The model under review builds one solid part; all positions refer to its coordinate system, in mm. Face numbers are marked on the shaded views. A direction names the side the tool comes from. Round coordinates to 2 decimals unless told otherwise and drop trailing zeros. Order: outer loops, then holes, each group sorted by start corner. A loop starts at its lowest first (then second) coordinate and runs counter-clockwise, first axis right, second up.
```python
from build123d import *

# Parameters (mm, degrees)
SKETCH1_W           = 40.25
SKETCH1_H           = 40
BOSS_EXTRUDE1_DEPTH = 20.25
SKETCH2_R           = 6.5
BOSS_EXTRUDE2_DEPTH = 1.35
SKETCH3_R           = 3
BOSS_EXTRUDE3_DEPTH = 4.25
BOSS_EXTRUDE4_DEPTH = 5.1


with BuildPart() as part:
    # Sketch1 → Boss-Extrude1 (new body)
    with BuildSketch(Plane(origin=(0, 0, 0), x_dir=(1, 0, 0), z_dir=(0, 1, 0))):
        with Locations((20.125, 20)):
            Rectangle(SKETCH1_W, SKETCH1_H)
    extrude(amount=BOSS_EXTRUDE1_DEPTH)

    # Sketch2 → Boss-Extrude2 (add)
    with BuildSketch(Plane.ZY):
        with Locations(Location((-29.5, 10.125, 0), (0, 0, 180))):
            Circle(SKETCH2_R)
    extrude(amount=BOSS_EXTRUDE2_DEPTH)

    # Sketch3 → Boss-Extrude3 (add)
    with BuildSketch(Plane.ZY.offset(1.35)):
        with Locations((-29.5, 10.125)):
            Circle(SKETCH3_R)
    extrude(amount=BOSS_EXTRUDE3_DEPTH)

    # Sketch4 → Boss-Extrude4 (add)
    with BuildSketch(Plane(origin=(12.65, 0, 0), x_dir=(0, 0, -1), z_dir=(1, 0, 0))):
        with BuildLine():
            Line((40, 19.25), (46, 19.25))
            ThreePointArc((46, 19.25), (46.707106781, 18.957106781), (47, 18.25))
            Line((47, 18.25), (47, 15.655745837))
            ThreePointArc((47, 15.655745837), (43.25, 14.6875), (47, 13.719254163))
            Line((47, 13.719254163), (47, 6.530745837))
            ThreePointArc((47, 6.530745837), (43.25, 5.5625), (47, 4.594254163))
            Line((47, 4.594254163), (47, 2))
            ThreePointArc((47, 2), (46.707106781, 1.292893219), (46, 1))
            Line((46, 1), (40, 1))
            Line((40, 1), (40, 19.25))
        make_face()
        with BuildLine():
            Line((0, 19.25), (-6, 19.25))
            ThreePointArc((-6, 19.25), (-6.707106781, 18.957106781), (-7, 18.25))
            Line((-7, 18.25), (-7, 15.655745837))
            ThreePointArc((-7, 15.655745837), (-3.25, 14.6875), (-7, 13.719254163))
            Line((-7, 13.719254163), (-7, 6.530745837))
            ThreePointArc((-7, 6.530745837), (-3.25, 5.5625), (-7, 4.594254163))
            Line((-7, 4.594254163), (-7, 2))
            ThreePointArc((-7, 2), (-6.707106781, 1.292893219), (-6, 1))
            Line((-6, 1), (0, 1))
            Line((0, 1), (0, 19.25))
        make_face()
    extrude(amount=-BOSS_EXTRUDE4_DEPTH)


solid = part.part
```
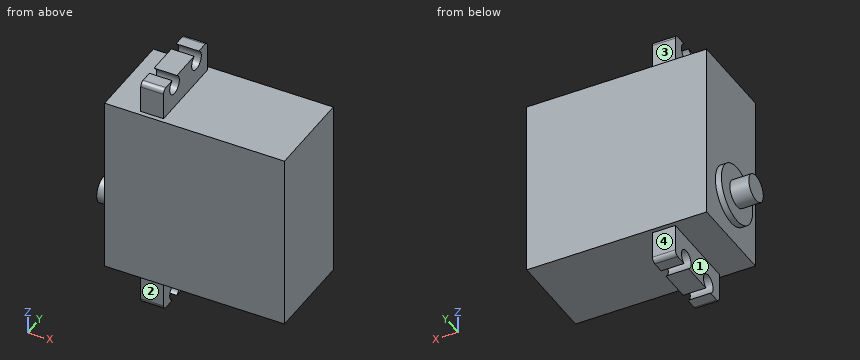
(1) Consider section D-D (x = 35). Write out the cut boundary in (y, z).
Data:
outline: (0, -40) - (20.25, -40) - (20.25, 0) - (0, 0) - close
(2) Insertion check: pin 1 (2.5 mm diameter, centred on x = 10, z = 2.5, fed in from -Y); pin 2 (6 mm diameter, centred on y = 10.5, z = -11, fed in from -X); pin 3 (10 mm diameter, centred on x = -1, y = 6.5, fed in from +Z). Each pin has a flat end and moves straight along its axis. Give the tip position at first contact, or say it passes through.
Data:
pin 1: stops at y = 1
pin 2: stops at x = 0
pin 3: stops at z = 0
(3) Consider section A-A (z = 5.25). Write out the cut boundary in (x, y).
Data:
outline: (7.55, 1) - (12.65, 1) - (12.65, 3.56) - (7.55, 3.56) - close; (7.55, 7.56) - (12.65, 7.56) - (12.65, 12.69) - (7.55, 12.69) - close; (7.55, 16.69) - (12.65, 16.69) - (12.65, 19.25) - (7.55, 19.25) - close
(4) Consider section C-C (y = 9.25). Write out the cut boundary in (x, z), and give its area (3 significant figures).
Data:
outline: (-5.6, -32.37) - (-1.35, -32.37) - (-1.35, -35.94) - (0, -35.94) - (0, -40) - (7.55, -40) - (7.55, -47) - (12.65, -47) - (12.65, -40) - (40.25, -40) - (40.25, 0) - (12.65, 0) - (12.65, 7) - (7.55, 7) - (7.55, 0) - (0, 0) - (0, -23.06) - (-1.35, -23.06) - (-1.35, -26.63) - (-5.6, -26.63) - close
area: 1,720 mm2
(5) For the marked faces 1, 2, 3 and 4, list the 3-axis set-ups (+Z, -Z, +X, -X, +Y, -Y) from which the entire face can be reached by the end or side of a thin tool; tool diameter is ignored.
Data:
face 1: -Z, -X, +Y, -Y
face 2: -Z, +X, -X, -Y
face 3: +Z, +X, -X, +Y
face 4: -Z, +X, -X, +Y
(6) Consider section B-B (z = -29.5). Write out the cut boundary in (x, y) (3 decimals).
Data:
outline: (-5.6, 7.125) - (-1.35, 7.125) - (-1.35, 3.625) - (0, 3.625) - (0, 0) - (40.25, 0) - (40.25, 20.25) - (0, 20.25) - (0, 16.625) - (-1.35, 16.625) - (-1.35, 13.125) - (-5.6, 13.125) - close
(7) To check wall thickness, follow probe 1 along Y at (x, z) = (11.65, -45.25); probe 2 along Y at (x, z) = (10, 5); probe 3 along Z at (x, y) = (36.5, 6). State the ranges of each line that lie inside material, in increasing order.
Data:
probe 1: y = 1 to 3.56, 7.56 to 12.69, 16.69 to 19.25
probe 2: y = 1 to 3.58, 7.55 to 12.7, 16.67 to 19.25
probe 3: z = -40 to 0
